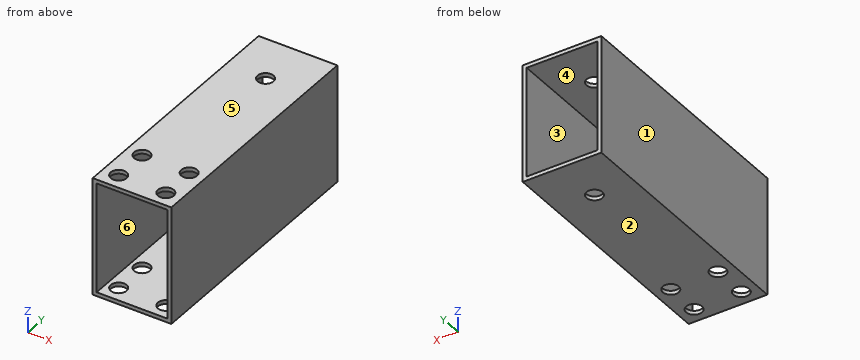
```python
from build123d import *

# Parameters (mm, degrees)
SKETCH_2_W               = 20
SKETCH_2_H               = 30
EXTRUDE_1_DEPTH          = 61.5
SKETCH_3_W               = 18
SKETCH_3_H               = 28
CUT_EXTRUDE_1_DEPTH      = 62.5
CUT_EXTRUDE_1_DEPTH_BACK = 62.5
SKETCH_4_W               = 30
SKETCH_4_H               = 45.05
CUT_EXTRUDE_2_DEPTH      = 21
SKETCH_5_R               = 2.025
CUT_EXTRUDE_3_DEPTH      = 31
SKETCH_6_W               = 20
SKETCH_6_H               = 14
CUT_EXTRUDE_4_DEPTH      = 1
CUT_EXTRUDE_4_DEPTH_BACK = 31
SKETCH_7_R               = 2.025
CUT_EXTRUDE_5_DEPTH      = 1
CUT_EXTRUDE_5_DEPTH_BACK = 31
SKETCH_8_R               = 2.025
CUT_EXTRUDE_6_DEPTH      = 31


with BuildPart() as part:
    # 草图2 → 凸台-拉伸1 (new body, symmetric)
    with BuildSketch(Plane(origin=(0, 0, 0), x_dir=(1, 0, 0), z_dir=(0, 1, 0))):
        Rectangle(SKETCH_2_W, SKETCH_2_H)
    extrude(amount=EXTRUDE_1_DEPTH, both=True)

    # 草图3 → 切除-拉伸1 (cut, two sides)
    with BuildSketch(Plane(origin=(0, 0, 0), x_dir=(1, 0, 0), z_dir=(0, 1, 0))) as cut_extrude_1_sk:
        Rectangle(SKETCH_3_W, SKETCH_3_H)
    extrude(amount=CUT_EXTRUDE_1_DEPTH, mode=Mode.SUBTRACT)
    extrude(cut_extrude_1_sk.sketch, amount=-CUT_EXTRUDE_1_DEPTH_BACK, mode=Mode.SUBTRACT)

    # 草图4 → 切除-拉伸2 (cut, through all)
    with BuildSketch(Plane.ZY.offset(10)):
        with Locations((0, 38.975)):
            Rectangle(SKETCH_4_W, SKETCH_4_H)
    extrude(amount=-CUT_EXTRUDE_2_DEPTH, mode=Mode.SUBTRACT)

    # 草图5 → 切除-拉伸3 (cut, through all)
    with BuildSketch(Plane.XY.offset(15)):
        with Locations((-6, -48.55)):
            Circle(SKETCH_5_R)
        with Locations((6, -48.55)):
            Circle(SKETCH_5_R)
    extrude(amount=-CUT_EXTRUDE_3_DEPTH, mode=Mode.SUBTRACT)

    # 草图6 → 切除-拉伸4 (cut, two sides)
    with BuildSketch(Plane.XY.offset(15)) as cut_extrude_4_sk:
        with Locations((0, 9.45)):
            Rectangle(SKETCH_6_W, SKETCH_6_H)
    extrude(amount=CUT_EXTRUDE_4_DEPTH, mode=Mode.SUBTRACT)
    extrude(cut_extrude_4_sk.sketch, amount=-CUT_EXTRUDE_4_DEPTH_BACK, mode=Mode.SUBTRACT)

    # 草图7 → 切除-拉伸5 (cut, two sides)
    with BuildSketch(Plane.XY.offset(15)) as cut_extrude_5_sk:
        with Locations((-6, -57.55)):
            Circle(SKETCH_7_R)
        with Locations((6, -57.55)):
            Circle(SKETCH_7_R)
    extrude(amount=CUT_EXTRUDE_5_DEPTH, mode=Mode.SUBTRACT)
    extrude(cut_extrude_5_sk.sketch, amount=-CUT_EXTRUDE_5_DEPTH_BACK, mode=Mode.SUBTRACT)

    # 草图8 → 切除-拉伸6 (cut, through all)
    with BuildSketch(Plane.XY.offset(15)):
        with Locations((0, -10.05)):
            Circle(SKETCH_8_R)
    extrude(amount=-CUT_EXTRUDE_6_DEPTH, mode=Mode.SUBTRACT)


solid = part.part
```
The listing builds one solid part. Answer for the finished solid, in the listing's coordinates (mm). Face numbers are marked on the shaded views. A direction names the side the tool comes from. Round coordinates to 2 decimals unless told otherwise and drop trailing zeros. Write each loop counter-clockwise with the first axis right and the second up, starting at its lowest first coordinate (ties: lowest second). Pieces come first, ordered by that corner, then holes. Notation, with made-up numbers: (-6, -38.5) -> (12, -38.5) arc R6 cw to (12, -29.5) -> close; hole circle Ø1 at (62.5, 47.25). An arc over 180 degrees is marked (long way). Answer as a JSON object with one key per item and string values. Group by question number.
Q1. Section B-B (x = 6) is taken. Write down the section's boundary in (y, z) (3 decimals), plus the area to 3 significant figures.
Q2. Section C-C (y = -10.05) is taken. Write down the section's boundary in (x, z) (3 decimals), plus the area to 3 significant figures.
Q3. Straight lines are drawn through the part: line 1 along Y through (x, z) = (6, -14.3) (3 decimals); line 2 along Z through (x, y) = (4.75, -21); line 3 along X through (y, z) = (-38.5, 10.5). For each, find the intervals that lie inside material, in ascending order.
Q4. Section D-D (y = -48.55) is taken. Write down the section's boundary in (x, z) (3 decimals), plus the area to 3 significant figures.
Q5. Determine the mould class of the marked faces 1, 2, 3 and 4 for opening direction Z: pulls with the +Z half, pulls with the -Z half, needs draft (parallel to the pull), parting line crosses it, or undercut.
Q6. Which of the six approach directions +Z, -Z, +X, -X, +Y, -Y give full straight-line access (tool end or side, diameter ignored) to the marked faces 5 and 6?
Q7. This flat-tipped pin is pushed along its axis until it touches: pin 1 Ø2.5 at (x, y) = (-6, -48.55) entering from +Z. Where does it stop, or does it pass through?
Q8. Section A-A (z = 1.25) is taken. Write down the section's boundary in (x, y), plus the area to 3 significant figures.
Check values:
{
 "1": {"outline": "(-61.5, -15) -> (-59.575, -15) -> (-59.575, -14) -> (-61.5, -14) -> close; (-61.5, 14) -> (-59.575, 14) -> (-59.575, 15) -> (-61.5, 15) -> close; (-55.525, -15) -> (-50.575, -15) -> (-50.575, -14) -> (-55.525, -14) -> close; (-55.525, 14) -> (-50.575, 14) -> (-50.575, 15) -> (-55.525, 15) -> close; (-46.525, -15) -> (2.45, -15) -> (2.45, -14) -> (-46.525, -14) -> close; (-46.525, 14) -> (2.45, 14) -> (2.45, 15) -> (-46.525, 15) -> close", "area": "112 mm^2"},
 "2": {"outline": "(-10, -15) -> (-2.025, -15) -> (-2.025, -14) -> (-9, -14) -> (-9, 14) -> (-2.025, 14) -> (-2.025, 15) -> (-10, 15) -> close; (2.025, -15) -> (10, -15) -> (10, 15) -> (2.025, 15) -> (2.025, 14) -> (9, 14) -> (9, -14) -> (2.025, -14) -> close", "area": "87.9 mm^2"},
 "3": {"line 1": "-61.5 to -59.575, -55.525 to -50.575, -46.525 to 2.45", "line 2": "-15 to -14, 14 to 15", "line 3": "-10 to -9, 9 to 10"},
 "4": {"outline": "(-10, -15) -> (-8.025, -15) -> (-8.025, -14) -> (-9, -14) -> (-9, 14) -> (-8.025, 14) -> (-8.025, 15) -> (-10, 15) -> close; (-3.975, -15) -> (3.975, -15) -> (3.975, -14) -> (-3.975, -14) -> close; (-3.975, 14) -> (3.975, 14) -> (3.975, 15) -> (-3.975, 15) -> close; (8.025, -15) -> (10, -15) -> (10, 15) -> (8.025, 15) -> (8.025, 14) -> (9, 14) -> (9, -14) -> (8.025, -14) -> close", "area": "79.8 mm^2"},
 "5": {"face 1": "needs draft", "face 2": "pulls with the -Z half", "face 3": "undercut", "face 4": "undercut"},
 "6": {"face 5": "+Z, +X, -X, +Y, -Y", "face 6": "+Y, -Y"},
 "7": {"pin 1": "through"},
 "8": {"outline": "(-10, -61.5) -> (-9, -61.5) -> (-9, 2.45) -> (-10, 2.45) -> close; (9, -61.5) -> (10, -61.5) -> (10, 2.45) -> (9, 2.45) -> close", "area": "128 mm^2"}
}
